Read the model definition and answer for the solid it produces. Units are mm, in the model's axes. Give positions to 0.01 mm unless a question says otherwise; leave off trailing zeros. Write each loop counter-clockwise with the first axis right and the second up, starting at its lowest first coordinate (ties: lowest second). Pieces come first, ordered by that corner, then holes. Notation, with made-up numbers: (-39, 56) - (-29, 56) arc R15 ccw to (-29, 77) - close; hole circle Ø10 at (80.25, 0.5). An arc over 180 degrees is marked (long way). Answer as a JSON object with one key per item and string values. Group by question number.
```python
from build123d import *

# Parameters (mm, degrees)
Y_KSEKLIK_EKSTR_ZYON1_DEPTH = 7.5
IZIM2_R                     = 9
KES_EKSTR_ZYON1_DEPTH       = 16


with BuildPart() as part:
    # Çizim1 → Yükseklik-Ekstrüzyon1 (new body, symmetric)
    with BuildSketch(Plane.XY):
        with BuildLine():
            Line((0, 0), (0, 135))
            Line((0, 135), (65, 110))
            Line((65, 110), (65, 84.393876913))
            ThreePointArc((65, 84.393876913), (53, 55), (65, 25.606123087))
            Line((65, 25.606123087), (65, 0))
            Line((65, 0), (0, 0))
        make_face()
    extrude(amount=Y_KSEKLIK_EKSTR_ZYON1_DEPTH, both=True)

    # Çizim2 → Kes-Ekstrüzyon1 (cut, through all)
    with BuildSketch(Plane.XY.offset(7.5)):
        with Locations((13, 100)):
            Circle(IZIM2_R)
        with Locations((13, 25)):
            Circle(IZIM2_R)
    extrude(amount=-KES_EKSTR_ZYON1_DEPTH, mode=Mode.SUBTRACT)


solid = part.part
```
1) Find the intervals of material crossed by line 1 (X direction, y = 99.5, z = 3); line 2 (Y direction, x = 13, z = 3.5); line 3 (X direction, y = 106, z = 1.75), in increasing order. Write a range as [from, to].
2) A flat-ended cylindrical pin translates along its axis: pin 1 Ø1.5 at (y, z) = (32.5, 1) entering from -X. Find the tip coordinate at first contact, or state that the pin passes through.
3) Find section A-A, the plane y = 100. Write down the section's boundary in (x, z), and give its area (3 significant figures).
4) For a pull along X with two mould halves and no side action, classify faces 1 (the flat face through (33, 0, 0)), 2 (the cylindrical face through (17.84, 32.59, 0.11)), 3 (the cylindrical face through (11.049, 91.214, 0.105)), 4 (the flat face through (32.045, 122.675, 0.105)) as released by +X, released by -X, zero draft, split by the parting line, or undercut.
5) Find section D-D, the plane x = 58.5. Write down the section's boundary in (y, z), and give its area (3 significant figures).
6) Find section C-C, the plane z = -6. Write down the section's boundary in (x, y), and give its area (3 significant figures).
7) Find section B-B, the plane x = 13. Write down the section's boundary in (y, z).
Values follow:
{
 "1": {"line 1": "x = [0, 4.01], [21.99, 65]", "line 2": "y = [0, 16], [34, 91], [109, 130]", "line 3": "x = [0, 6.29], [19.71, 65]"},
 "2": {"pin 1": "stops at x = 0"},
 "3": {"outline": "(0, -7.5) - (4, -7.5) - (4, 7.5) - (0, 7.5) - close; (22, -7.5) - (65, -7.5) - (65, 7.5) - (22, 7.5) - close", "area": "705 mm2"},
 "4": {"face 1": "zero draft", "face 2": "undercut", "face 3": "undercut", "face 4": "released by +X"},
 "5": {"outline": "(0, -7.5) - (34.22, -7.5) - (34.22, 7.5) - (0, 7.5) - close; (75.78, -7.5) - (112.5, -7.5) - (112.5, 7.5) - (75.78, 7.5) - close", "area": "1,060 mm2"},
 "6": {"outline": "(0, 0) - (65, 0) - (65, 25.61) arc R42 cw to (65, 84.39) - (65, 110) - (0, 135) - close; hole circle Ø18 at (13, 25); hole circle Ø18 at (13, 100)", "area": "6,970 mm2"},
 "7": {"outline": "(0, -7.5) - (16, -7.5) - (16, 7.5) - (0, 7.5) - close; (34, -7.5) - (91, -7.5) - (91, 7.5) - (34, 7.5) - close; (109, -7.5) - (130, -7.5) - (130, 7.5) - (109, 7.5) - close"}
}
